Autodesk Fusion 360 part; units mm, degrees
sketch "Sketch1" plane through (0, 0, 0) normal (0, 1, 0) x (1, 0, 0)
  line L0 (0, 0) -> (76.2, 0)
  line L1 (76.2, 0) -> (76.2, -203.2)
  line L2 (76.2, -203.2) -> (0, -203.2)
  line L3 (0, -203.2) -> (0, 0)
  dimension "d1" = 76.2
  dimension "d2" = 203.2
sketch "Sketch2" plane through (0, 50, 0) normal (0, 1, 0) x (-1, 0, 0)
  line L0 (0, 203.2) -> (-76.2, 203.2)
  line L1 (-76.2, 203.2) -> (-76.2, 0)
  line L2 (-76.2, 0) -> (0, 0)
  line L3 (0, 0) -> (0, 203.2)
  line L4 (150, 0) -> (73.8, 0)
  line L5 (73.8, 0) -> (73.8, 127)
  line L6 (73.8, 127) -> (150, 127)
  line L7 (150, 127) -> (150, 0)
  dimension "d8" = 76.2
  dimension "d9" = 127
extrude "Extrude2" add sketch "Sketch2" along normal blind 76.2 contours L4 L5 L6 L7
shell "Shell1" thickness 3.81 removed faces 1 at (-99.2, 126.2, 42.3333)
sketch "Sketch3" plane through (0, 0, 0) normal (0, 1, 0) x (1, 0, 0)
  line L0 (79.4367, 34.7313) -> (3.2367, 34.7313)
  line L1 (3.2367, 34.7313) -> (3.2367, 237.9313)
  line L2 (3.2367, 237.9313) -> (79.4367, 237.9313)
  line L3 (79.4367, 237.9313) -> (79.4367, 34.7313)
  dimension "d13" = 76.2
  dimension "d14" = 203.2
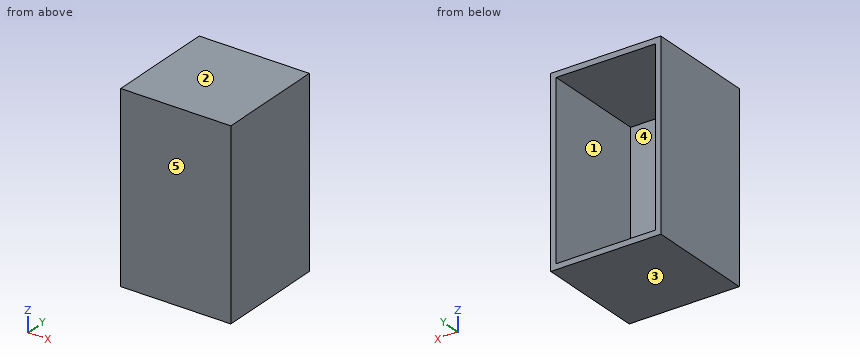
The model under review builds one solid part; all positions refer to its coordinate system, in mm. Face numbers are marked on the shaded views. A direction names the side the tool comes from. Give positions to 0.01 mm unless a question says otherwise; leave off trailing zeros. Write each loop counter-clockwise with the first axis right and the second up, starting at its lowest first coordinate (ties: lowest second). Pieces come first, ordered by that corner, then holes. Notation, with made-up numbers: (50.25, 15.5) -> (55.25, 15.5) arc R17 cw to (55.25, 46.5) -> close; hole circle Ø7 at (-17.5, 22). An arc over 180 degrees is marked (long way). Answer in a Markdown table with one row per item.
1) Add section A-A on z = 48.5. State the section outline as (x, y) points.
Worked answers:
| item | result |
|---|---|
| outline | (-150, 50) -> (-73.8, 50) -> (-73.8, 126.2) -> (-77.61, 126.2) -> (-77.61, 53.81) -> (-146.19, 53.81) -> (-146.19, 126.2) -> (-150, 126.2) -> close |
2) For L1, parallel to Z at x = -90.5, y = 105; L2, parallel to X at y = 62.5, z = 104; L3, parallel to Y at x = -126.5, z = 45.5, list the stretches that pass through material, from the lowest coordinate up. Write a range as [from, to].
Worked answers:
| item | result |
|---|---|
| L1 | [0, 3.81], [123.19, 127] |
| L2 | [-150, -146.19], [-77.61, -73.8] |
| L3 | [50, 53.81] |
3) Tool access review of the marked faces 1 and 2: name each direction out of +Z, -Z, +X, -X, +Y, -Y from which nothing blocks a thin tool from reaching the whole face with its end or side.
Worked answers:
| item | result |
|---|---|
| face 1 | +Y |
| face 2 | +Z, +X, -X, +Y, -Y |
4) Add section B-B on y = 120.5. State the section outline as (x, z) points, plus the area to 3 significant figures.
Worked answers:
| item | result |
|---|---|
| outline | (-150, 0) -> (-73.8, 0) -> (-73.8, 127) -> (-150, 127) -> close; hole (-146.19, 3.81) -> (-77.61, 3.81) -> (-77.61, 123.19) -> (-146.19, 123.19) -> close |
| area | 1,490 mm² |
5) Mouldability with a two-part tool opening along Y and no side actions: class the marked faces 3, 4 and 5 as +Y half, -Y half, draft (parallel to the pull), parting line (faces both ways), or undercut.
Worked answers:
| item | result |
|---|---|
| face 3 | draft |
| face 4 | +Y half |
| face 5 | -Y half |
6) Add section C-C on x = -111. State the section outline as (y, z) points.
Worked answers:
| item | result |
|---|---|
| outline | (50, 0) -> (126.2, 0) -> (126.2, 3.81) -> (53.81, 3.81) -> (53.81, 123.19) -> (126.2, 123.19) -> (126.2, 127) -> (50, 127) -> close |
7) Clearance check with a flat-ended pin moving along its axis: P1, Ø12, axis at x = -118.5, z = 91.5, coming from the +Y side. State where the tip first meets the part, or that it passes through.
Worked answers:
| item | result |
|---|---|
| P1 | y = 53.81 |
